Autodesk Inventor part; units mm, degrees
ref_plane "YZ Plane" through (0, 0, 0) normal (1, 0, 0) x (0, 1, 0)
ref_plane "XZ Plane" through (0, 0, 0) normal (0, 1, 0) x (-1, 0, 0)
ref_plane "XY Plane" through (0, 0, 0) normal (0, 0, 1) x (1, 0, 0)
sketch "Sketch1" plane through (0, 0, 0) normal (0, 0, 1) x (1, 0, 0)
  line L0 (0, -3.175) -> (25.4, -3.175)
  arc A0 (25.4, -3.175) -> (25.4, 3.175) centre (25.4, 0) ccw
  line L1 (25.4, 3.175) -> (0, 3.175)
  arc A1 (0, 3.175) -> (0, -3.175) centre (0, 0) ccw
  arc A2 (0, 9.525) -> (0, -9.525) centre (0, 0) ccw
  line L2 (0, 9.525) -> (28.575, 9.525)
  line L3 (0, -9.525) -> (28.575, -9.525)
  arc A3 (28.575, 9.525) -> (38.1, 19.05) centre (28.575, 19.05) ccw
  arc A4 (38.1, -19.05) -> (28.575, -9.525) centre (28.575, -19.05) ccw
  line L4 (38.1, -19.05) -> (63.5, -19.05)
  line L5 (38.1, 19.05) -> (63.5, 19.05)
  line L6 (44.45, 15.875) -> (57.15, 15.875)
  line L7 (53.975, 9.525) -> (53.975, -9.525)
  line L8 (47.625, -9.525) -> (47.625, 9.525)
  arc A5 (53.975, 9.525) -> (47.625, 9.525) centre (50.8, 9.525) ccw
  line L9 (44.45, 15.875) -> (44.45, -15.875)
  line L10 (44.45, -15.875) -> (57.15, -15.875)
  line L11 (57.15, 15.875) -> (57.15, -15.875)
  arc A6 (47.625, -9.525) -> (53.975, -9.525) centre (50.8, -9.525) ccw
  line L12 (-24.13, 0) -> (78.105, 0)
  line L13 (0, -26.67) -> (0, 26.67)
  line L14 (63.5, 19.05) -> (63.5, -19.05)
  point P0 (0, 0)
  point P1 (50.8, 12.7)
  point P2 (50.8, 15.875)
  point P3 (50.8, 19.05)
  point P4 (50.8, -19.05)
  point P5 (63.5, 0)
  point P6 (47.625, 0)
  point P7 (53.975, 0)
  point P8 (44.45, 0)
  point P9 (57.15, 0)
  dimension "d25" = 63.5
  dimension "d26" = 25.4
  dimension "d27" = 6.35
  dimension "d28" = 12.7
  dimension "d29" = 3.175
  dimension "d30" = 9.525
  dimension "d31" = 3.175
  dimension "d32" = 25.4
  dimension "d33" = 38.1
  dimension "d34" = 3.175
  dimension "d35" = 19.05
  dimension "d36" = 31.75
extrude "Extrusion1" add sketch "Sketch1" along normal blind 3.175 contours L13 L12 A0 L0 | L13 A2 L12 A1 | L0 A0 L12 L9 L10 L11 L14 L4 A4 L3 L13 | A1 L12 L13 | L12 A2 L13 A1 | A1 L13 L12 | L13 L1 A0 L12 | A0 L1 L13 L2 A3 L5 L14 L12 L11 L6 L9
extrude "Extrusion2" add sketch "Sketch1" along normal blind 6.35 contours L12 L8 A6 L7 L11 L10 L9 | L9 L6 L11 L12 L7 A5 L8
sketch "Sketch2" plane through (0, 0, 3.175) normal (0, 0, 1) x (1, 0, 0)
  circle A0 centre (0, 0) radius 3.175
  line L0 (0, 3.175) -> (25.4, 3.175)
  circle A1 centre (25.4, 0) radius 3.175
  line L1 (0, -3.175) -> (25.4, -3.175)
  line L2 (-24.13, 0) -> (78.105, 0)
  dimension "d37" = 6.35
  dimension "d38" = 25.4
extrude "Extrusion3" cut sketch "Sketch2" against normal through all
properties part number "Ch3 Part 1"
Check sheet for the modelled part. Datum: model origin and axes. Units: mm. A direction names the side the tool comes from. Give positions to 0.01 mm unless a question says otherwise; leave off trailing zeros. Order: outer loops, then holes, each group sorted by start corner. A loop starts at its lowest first (then second) coordinate and runs counter-clockwise, first axis right, second up. Notation, with made-up numbers: M -13.5,-4.75 L 26.5,-4.75 A25 cw 26.5,27.25 Z; hole C 3.25,54 d5. An arc over 180 degrees is marked long. Answer in a Markdown table with one row per item. Add a question column.
Q1. Sectioned sample at D-D, the plane y = -11. Record the boundary of the cut face in (x, z) (3 decimals).
Q2. Release check for a two-part mould opening along X. For faces 1 (the cylindrical face through (35.236, -12.241, 1.565)), 2 (the flat face through (63.5, 0, 2)), 3 (the cylindrical face through (50.9, -12.7, 3.1)) record: released by +X, released by -X, zero draft, split by the parting line, or undercut.
Q3. Thickness scan on L1, parallel to X at y = 7.5, z = 4.25 (3 decimals); L2, parallel to Y at x = 23, z = 1 (3 decimals); L3, parallel to Z at x = 58, y = 17.5 (3 decimals). Record the ranges inside material, lowest first.
Q4. Sectioned sample at B-B, the plane y = 0. Record the boundary of the cut face in (x, z) (3 decimals), and give its area (3 significant figures).
Q5. Access from +Z, -Z, +X, -X, +Y, -Y to the whole of each face (thin tool, end or side, straight path). Record for faces 4 (the flat face through (47.625, 0, 3)), 5 (the flat face through (57.15, 0, 5)), 6 (the flat face through (14, -9.525, 2)).
Q6. Sectioned sample at C-C, the plane z = 2. Record the boundary of the cut face in (x, y) (3 decimals).
Q7. Gauge pin test, flat ends, axial feed: pin 1 Ø1.6 at (x, z) = (21, 1.5) entering from -Y (3 decimals); pin 2 Ø6 at (x, y) = (16.5, -4) entering from +Z (3 decimals); pin 3 Ø2.5 at (x, z) = (11, 1) entering from +Y (3 decimals); pin 4 Ø1.5 at (x, z) = (24, 4) entering from +Y. Record the tip position at first contact, or that the pin passes through.
Q8. Sectioned sample at A-A, the plane x = 23. Record the boundary of the cut face in (y, z) (3 decimals).
Verdict:
| question | item | result |
|---|---|---|
| 1 | outline | M 33.666,0 L 47.988,0 L 47.988,6.35 L 44.45,6.35 L 44.45,3.175 L 33.666,3.175 Z; M 53.612,0 L 63.5,0 L 63.5,3.175 L 57.15,3.175 L 57.15,6.35 L 53.612,6.35 Z |
| 2 | face 1 | released by -X |
| 2 | face 2 | released by +X |
| 2 | face 3 | undercut |
| 3 | L1 | 44.45 to 47.625, 53.975 to 57.15 |
| 3 | L2 | -9.525 to -3.175, 3.175 to 9.525 |
| 3 | L3 | 0 to 3.175 |
| 4 | outline | M -9.525,0 L -3.175,0 L -3.175,3.175 L -9.525,3.175 Z; M 28.575,0 L 47.625,0 L 47.625,6.35 L 44.45,6.35 L 44.45,3.175 L 28.575,3.175 Z; M 53.975,0 L 63.5,0 L 63.5,3.175 L 57.15,3.175 L 57.15,6.35 L 53.975,6.35 Z |
| 4 | area | 131 mm² |
| 5 | face 4 | +Z, -Z |
| 5 | face 5 | +Z, +X, +Y, -Y |
| 5 | face 6 | +Z, -Z, -X, -Y |
| 6 | outline | M 0,-9.525 L 28.575,-9.525 A9.525 cw 38.1,-19.05 L 63.5,-19.05 L 63.5,19.05 L 38.1,19.05 A9.525 cw 28.575,9.525 L 0,9.525 A9.525 ccw Z; hole M 0,-3.175 L 25.4,-3.175 A3.175 ccw 25.4,3.175 L 0,3.175 A3.175 ccw Z; hole M 47.625,-9.525 A3.175 ccw 53.975,-9.525 L 53.975,9.525 A3.175 ccw 47.625,9.525 Z |
| 7 | pin 1 | y = -9.525 |
| 7 | pin 2 | z = 3.175 |
| 7 | pin 3 | y = 9.525 |
| 7 | pin 4 | through |
| 8 | outline | M -9.525,0 L -3.175,0 L -3.175,3.175 L -9.525,3.175 Z; M 3.175,0 L 9.525,0 L 9.525,3.175 L 3.175,3.175 Z |
